Can you work these out from the model? Positions are in its coordinate system, mm. A direction names the side the tool comes from. Give positions to 0.01 mm unless a question says otherwise; leave off trailing zeros. Loops run counter-clockwise (first coordinate to the right, second up) from the corner with the lowest first, then second, coordinate; pieces in that order, holes last.
from build123d import *

# Parameters (mm, degrees)
FILLET_1_R          = 1
CHAMFER_1_SIZE      = 0.5
CHAMFER_2_SIZE      = 2
SKETCH_4_W          = 5
SKETCH_4_H          = 8.5
CUT_EXTRUDE_1_DEPTH = 30
CUT_EXTRUDE_2_DEPTH = 80.669630349


with BuildPart() as part:
    # 草图1 → 旋转1 (revolve)
    with BuildSketch(Plane(origin=(0, 0, 0), x_dir=(0, 0, -1), z_dir=(1, 0, 0))):
        Polygon((0, 0), (0, 14.5), (7, 14.5), (7, 12.5), (56, 12.5), (56, 10.795768266), (76, 10.795768266), (76, 0), align=None)
    revolve(axis=Axis((0, 0, -76), (0, 0, 1)))

    # 草图3 → 切除-旋转1 (revolve, cut)
    with BuildSketch(Plane(origin=(0, 0, 0), x_dir=(0, 0, -1), z_dir=(1, 0, 0))):
        Polygon((0, 0), (0, 7), (33.5, 7), (33.5, 2.75), (76, 2.75), (76, 0), align=None)
    revolve(axis=Axis((0, 0, -76), (0, 0, 1)), mode=Mode.SUBTRACT)

    # 圆角1
    fillet_1_edges = [part.edges().sort_by_distance(p)[0] for p in [
        (0, -7, -33.5),
    ]]
    fillet(fillet_1_edges, radius=FILLET_1_R)

    # 倒角1
    chamfer_1_edges = [part.edges().sort_by_distance(p)[0] for p in [
        (0, -7, 0),
        (0, -2.75, -33.5),
        (0, -2.75, -76),
        (0, -10.795768266, -76),
        (0, -14.5, -7),
        (0, -14.5, 0),
    ]]
    chamfer(chamfer_1_edges, length=CHAMFER_1_SIZE)

    # 倒角2
    # the kernel refuses this chamfer: 2 mm, written as the material it takes off along each edge
    with BuildSketch(Plane(origin=(0, 0, -56), x_dir=(0, 1, 0), z_dir=(1, 0, 0))) as chamfer_2_piece_1_section:
        Polygon((12.5, CHAMFER_2_SIZE), (12.5 - CHAMFER_2_SIZE, 0), (12.5, 0), align=None)
    chamfer_2_piece_1 = revolve(axis=Axis((0, 0, -56), (0, 0, 1)), mode=Mode.PRIVATE)
    chamfer_2_piece_1 = chamfer_2_piece_1 - Plane(origin=(0, 0, -54.862135047), x_dir=(0, 1, 0), z_dir=(0, 0, -1)) * Cylinder(10.795768266, 50, mode=Mode.PRIVATE)
    add(chamfer_2_piece_1, mode=Mode.SUBTRACT)

    # 草图4 → 切除-拉伸1 (cut)
    with BuildSketch(Plane.XY):
        with Locations((0, 4.25)):
            Rectangle(SKETCH_4_W, SKETCH_4_H)
    extrude(amount=-CUT_EXTRUDE_1_DEPTH, mode=Mode.SUBTRACT)

    # 草图5 → 切除-拉伸2 (cut, through all)
    with BuildSketch(Plane(origin=(0, 4.5, 0), x_dir=(1, 0, 0), z_dir=(0, 1, 0))):
        with BuildLine():
            Line((2.647884133, 72.852115867), (2.647884133, 58.352115867))
            ThreePointArc((2.647884133, 58.352115867), (0, 55.704231734), (-2.647884133, 58.352115867))
            Line((-2.647884133, 58.352115867), (-2.647884133, 72.852115867))
            ThreePointArc((-2.647884133, 72.852115867), (0, 75.5), (2.647884133, 72.852115867))
        make_face()
    extrude(amount=CUT_EXTRUDE_2_DEPTH, mode=Mode.SUBTRACT)


solid = part.part
(1) Suppose I cut it at B-B on z = -13. List the corners of the cut face in (x, y) for me, plus the area to 3 significant figures.
Returned:
outline: circle Ø25 at (0, 0); hole (-2.5, 6.54) arc R7 ccw (long way) to (2.5, 6.54) - (2.5, 8.5) - (-2.5, 8.5) - close
area: 329 mm2
(2) Thinking about a two-plate mould opening in Z: for faces 4 (the conical face through (-0.28, -7.137, -0.358)), 5 (the flat face through (0, 8.5, -15)), 6 (the flat face through (2.648, 7, -66)), which applies, pulls with the +Z half, pulls with the -Z half, needs draft (parallel to the pull), parting line crosses it, or undercut?
Returned:
face 4: pulls with the +Z half
face 5: needs draft
face 6: undercut
(3) Please list where these lines run through material, in increasing order: probe 1 along Y at (x, z) = (0, -54); probe 2 along X at (y, z) = (0, -25); probe 3 along Y at (x, z) = (0, -22).
Returned:
probe 1: y = -12.5 to -2.75, 2.75 to 12.5
probe 2: x = -12.5 to -7, 7 to 12.5
probe 3: y = -12.5 to -7, 8.5 to 12.5
(4) Will these pins go through, and if not, where does the flat tip stop? P1, Ø10, axis at y = -0.5, z = -52.5, coming from the -X side; P2, Ø6, axis at x = -1, y = 0.5, coming from the +Z side; P3, Ø2, axis at y = 8, z = -19.5, coming from the -X side.
Returned:
P1: stops at x = -12.5
P2: stops at z = -33.5
P3: stops at x = -10.36
(5) Which directions (+Z, -Z, +X, -X, +Y, -Y) give clear straight access to the entire face, cutting with the end or side of a thin tool? Please do faces 1 (the flat face through (2.5, 8, -15)), 2 (the cylindrical face through (-10.704, -1.405, -65.741)), 3 (the cylindrical face through (-0.1, 7.6, -75.5)).
Returned:
face 1: +Z
face 2: -Z
face 3: +Y
